Input: dimensioned drawing with shaded views. Units: mm. Origin: part minimum x, y, z. Give positions to 0.01 mm unless a question says otherwise; leave off trailing zeros. Loops run counter-clockwise (first coordinate to the right, second up) from the corner with the lowest first, then second, coordinate; pieces in that order, holes last. Notation, with made-up numbers: M 78.25,-30 L 114.25,-30 A9 ccw 114.25,-13 Z; hole C 38.5,2 d4. An arc over 180 degrees is marked long. Answer in a Markdown table with one row per item.
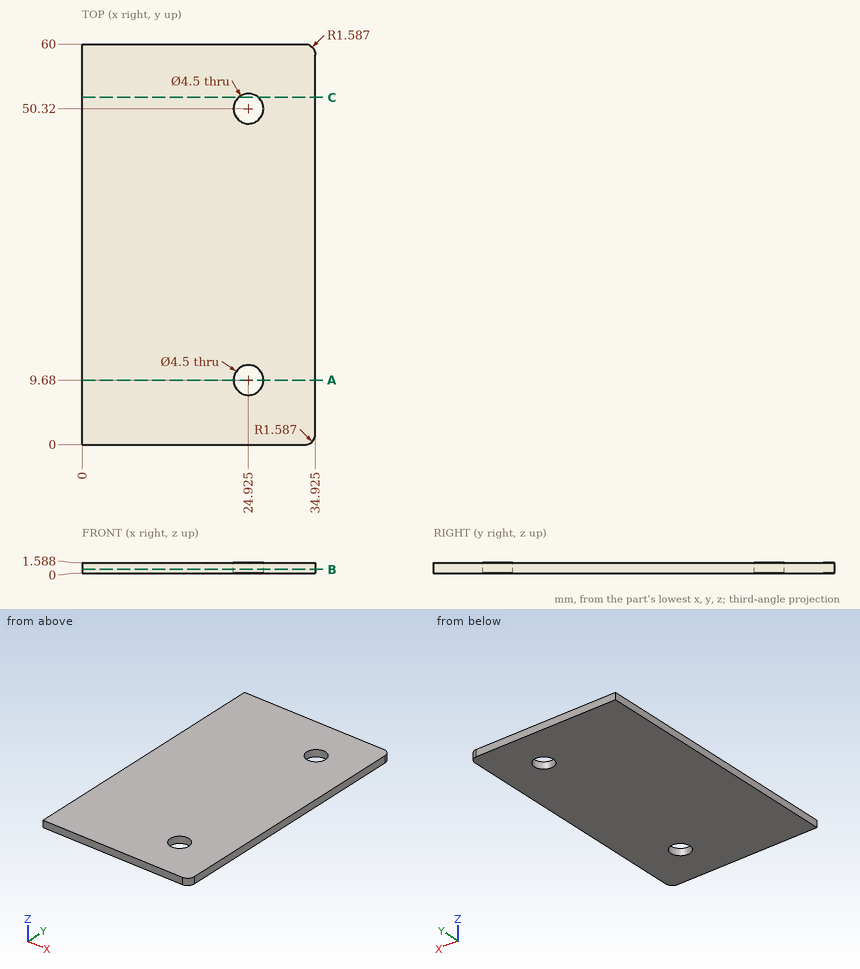
Q1. Ray query, probe 1 along Y at (x, z) = (26.5, 1.2) (1 decimal); probe 2 along Y at (x, z) = (25.5, 0.9) (1 decimal). Return the intervals inside material, ascending. Write a range as from..to.
Values follow:
| item | result |
|---|---|
| probe 1 | 0..8.1, 11.3..48.7, 51.9..60 |
| probe 2 | 0..7.5, 11.9..48.1, 52.5..60 |
Q2. Section query C-C (y = 52). Output: boundary loops of the cut face in (x, z) (1 decimal).
Values follow:
| item | result |
|---|---|
| outline | M 0,0 L 23.4,0 L 23.4,1.6 L 0,1.6 Z; M 26.4,0 L 34.9,0 L 34.9,1.6 L 26.4,1.6 Z |
Q3. Section query B-B (z = 0.6). Give the number of separate pieces and of enclosed holes in the cut face, plus the area to 3 significant figures.
Values follow:
| item | result |
|---|---|
| separate pieces | 1 |
| enclosed holes | 2 |
| area | 2,060 mm^2 |
Q4. Section query A-A (y = 9.68). Output: boundary loops of the cut face in (x, z) (1 decimal).
Values follow:
| item | result |
|---|---|
| outline | M 0,0 L 22.7,0 L 22.7,1.6 L 0,1.6 Z; M 27.2,0 L 34.9,0 L 34.9,1.6 L 27.2,1.6 Z |
